Input: part model. Units: mm. Frame: model coordinates. Face numbers are marked on the shaded views. Round coordinates to 2 decimals unless told otherwise and drop trailing zeros. Write each loop counter-clockwise with the first axis right and the second up, starting at its lowest first coordinate (ties: lowest second). Pieces come first, ordered by that corner, then holes. Notation, with made-up numbers: (8.25, 74.5) - (36.25, 74.5) arc R32 cw to (36.25, 105.5) - close; hole circle Ø5 at (-35.5, -18). An arc over 180 degrees is marked (long way). One line per item, written item: value. Start each with the question number.
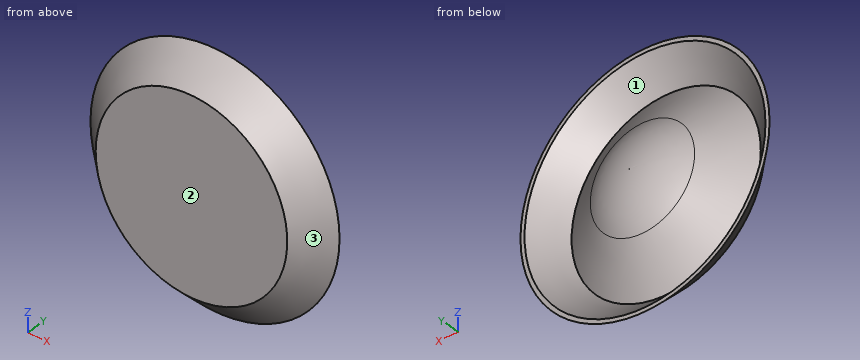
Autodesk Inventor part; units mm, degrees
ref_plane "Work Plane1" through (0, 15, 0) normal (0, 1, 0) x (-1, 0, 0)
ref_plane "Work Plane2" through (0, 25, 0) normal (0, 1, 0) x (1, 0, 0)
ref_plane "YZ Plane" through (0, 0, 0) normal (1, 0, 0) x (0, 1, 0)
sketch "Sketch1" plane through (0, 0, 0) normal (0, 1, 0) x (-1, 0, 0)
  circle A0 centre (0, 0) radius 50
  dimension "d0" = 100
ref_plane "Work Plane1" through (0, 15, 0) normal (0, 1, 0) x (-1, 0, 0)
sketch "Sketch2" plane through (0, 15, 0) normal (0, 1, 0) x (-1, 0, 0)
  circle A0 centre (0, 0) radius 65
  dimension "d2" = 130
loft "Loft1" add profiles "Sketch2", "Sketch1"
shell "Shell1" thickness 1.5 removed faces 1 at (7.4104, 15, 20.36)
ref_plane "Work Plane2" through (0, 25, 0) normal (0, 1, 0) x (1, 0, 0)
sketch "Sketch3" plane through (0, 25, 0) normal (0, 1, 0) x (1, 0, 0)
  circle A0 centre (0, 0) radius 15
  dimension "d9" = 30
loft "Loft2" add profiles "Sketch3" section 1 edges at (49.3787, 1.5, 0)
fillet "Fillet1" radius 48 1 edges at (15, 25, 0)
properties part number "Wadah"
Q1. Pull-direction query (Z, two-part tool) for the marked faces 1, 2 and 3; classes: pulls with the +Z half, pulls with the -Z half, needs draft (parallel to the pull), parting line crosses it, or undercut.
Q2. Material intervals for probe 1 along X at (y, z) = (10.5, -27.5); probe 2 along X at (y, z) = (13.5, -8.5); probe 3 along X at (y, z) = (9.75, 37.5), sorted ascending. Write a range as from..to.
Q3. Cut plane A-A, the plane y = 13.5. Output: boundary loops of the cut face in (x, z), and give its area (3 significant figures).
Q4. Contact query for flat-ended pins moving along their axis: pin 1 Ø8 at (y, z) = (5, -16.5) entering from -X; pin 2 Ø1 at (y, z) = (11, -32.5) entering from +X; pin 3 Ø5 at (x, y) = (34.5, 13.5) entering from -Z; pin 4 Ø8 at (x, z) = (2.5, 48.5) entering from -Y. Output: stop coordinate, or through.
A:
1. face 1: undercut
1. face 2: needs draft
1. face 3: parting line crosses it
2. probe 1: x = -53.89..-51.5, -23.56..23.56, 51.5..53.89
2. probe 2: x = -62.93..-60.79, -30.67..30.67, 60.79..62.93
2. probe 3: x = -46.52..-43.76, 43.76..46.52
3. outline: circle Ø127 at (0, 0); circle Ø63.65 at (0, 0); hole circle Ø122.76 at (0, 0)
3. area: 4,010 mm²
4. pin 1: stops at x = -56.8
4. pin 2: stops at x = 52.29
4. pin 3: stops at z = -56.29
4. pin 4: stops at y = 0
